from build123d import *

# Parameters (mm, degrees)
EXTRUDE_3_DEPTH          = 74.4
CUT_EXTRUDE_1_DEPTH      = 30
FILLET_1_R               = 5
CUT_EXTRUDE_6_DEPTH      = 330.484992071
CUT_EXTRUDE_6_DEPTH_BACK = 330.484992071
SKETCH_13_R              = 1.25
CUT_EXTRUDE_7_DEPTH      = 330.484992071
CUT_EXTRUDE_7_DEPTH_BACK = 330.484992071
SKETCH_14_R              = 2
SKETCH_15_R              = 2.5
CUT_EXTRUDE_8_DEPTH      = 100


with BuildPart() as part:
    # 草图4 → 凸台-拉伸3 (new body)
    with BuildSketch(Plane(origin=(0, 0, 0), x_dir=(0, 0, -1), z_dir=(1, 0, 0))):
        with BuildLine():
            Line((-19.997222801, -0.333287047), (-14.997222801, -300.333287047))
            ThreePointArc((-14.997222801, -300.333287047), (5.333287047, -319.997222801), (24.997222801, -299.666712953))
            Line((24.997222801, -299.666712953), (19.997222801, 0.333287047))
            ThreePointArc((19.997222801, 0.333287047), (-0.333287047, 19.997222801), (-19.997222801, -0.333287047))
        make_face()
    extrude(amount=EXTRUDE_3_DEPTH)

    # 草图8 → 切除-拉伸1 (cut)
    with BuildSketch(Plane(origin=(74.4, 0, 0), x_dir=(0, 0, -1), z_dir=(1, 0, 0))):
        with BuildLine():
            Line((-15.947486862, -243.317443397), (24.058068308, -243.317443397))
            Line((24.058068308, -243.317443397), (24.997222801, -299.666712953))
            ThreePointArc((24.997222801, -299.666712953), (4.858283924, -320.480273081), (-15.947486862, -300.333287047))
            Line((-15.947486862, -300.333287047), (-15.947486862, -243.317443397))
        make_face()
    extrude(amount=-CUT_EXTRUDE_1_DEPTH, mode=Mode.SUBTRACT)

    # 圆角1
    fillet_1_edges = [part.edges().sort_by_distance(p)[0] for p in [
        (74.4, -121.492078175, -22.027645554),
        (74.4, -243.317443397, -4.055290723),
        (74.4, 19.997222801, 0.333287047),
        (74.4, -121.825365222, 17.972354831),
    ]]
    fillet(fillet_1_edges, radius=FILLET_1_R)

    # 草图13 → 切除-拉伸6 (cut, two sides: drawn at the far end of the back side and taken through both)
    with BuildSketch(Plane.ZY.offset(-CUT_EXTRUDE_6_DEPTH_BACK)):
        with Locations(Location((-5.333287046, -270.358832161, 0), (0, 0, 180))):
            Circle(SKETCH_13_R)
        with Locations(Location((5.492030501, -276.608832161, 0), (0, 0, 180))):
            Circle(SKETCH_13_R)
        with Locations(Location((5.492030501, -289.108832161, 0), (0, 0, 180))):
            Circle(SKETCH_13_R)
        with Locations(Location((-5.333287046, -295.358832161, 0), (0, 0, 180))):
            Circle(SKETCH_13_R)
        with Locations(Location((-16.158604593, -289.108832161, 0), (0, 0, 180))):
            Circle(SKETCH_13_R)
        with Locations(Location((-16.158604593, -276.608832161, 0), (0, 0, 180))):
            Circle(SKETCH_13_R)
    extrude(amount=CUT_EXTRUDE_6_DEPTH + CUT_EXTRUDE_6_DEPTH_BACK, mode=Mode.SUBTRACT)

    # 草图14 → 切除-拉伸7 (cut, two sides: drawn at the far end of the back side and taken through both)
    with BuildSketch(Plane.ZY.offset(-CUT_EXTRUDE_7_DEPTH_BACK)):
        with Locations(Location((-5.333287046, -282.858832161, 0), (0, 0, 180))):
            Circle(SKETCH_14_R)
    extrude(amount=CUT_EXTRUDE_7_DEPTH + CUT_EXTRUDE_7_DEPTH_BACK, mode=Mode.SUBTRACT)

    # 草图15 → 切除-拉伸8 (cut)
    with BuildSketch(Plane.ZY):
        Circle(SKETCH_15_R)
    extrude(amount=-CUT_EXTRUDE_8_DEPTH, mode=Mode.SUBTRACT)


solid = part.part
The listing builds one solid part. Answer for the finished solid, in the listing's coordinates (mm). A direction names the side the tool comes from. Round coordinates to 2 decimals unless told otherwise and drop trailing zeros. Order: outer loops, then holes, each group sorted by start corner. A loop starts at its lowest first (then second) coordinate and runs counter-clockwise, first axis right, second up. Notation, with made-up numbers: (-32, 5) - (-15, 5) arc R22 cw to (-15, 27) - close; hole circle Ø3 at (78.25, 64). An arc over 180 degrees is marked (long way). Write item = value, one per line. Start each with the question number.
1) Given pin 1 (1.5 mm diameter, centred on y = -289.11, z = -16.16, fed in from +X); pin 2 (4 mm diameter, centred on x = 61, z = 9, fed in from -Y); pin 3 (3 mm diameter, centred on y = -270.36, z = -5.33, fed in from -X); pin 4 (1.5 mm diameter, centred on x = 34, z = 0.5, fed in from -Y), each flat-ended and moving along its own axis, determine where each tip first touches the part or whether it passes through.
2) For faces 1 (the flat face through (0, -148, -2)), 2 (the cylindrical face through (72.974, -123.501, 16.441)), 3 (the flat face through (57, -243.317, -4)), 4 (the cylindrical face through (72.97, -119.81, -20.5)), 5 (the flat face through (74.4, -110, -2)), determine the directions among +Z, -Z, +X, -X, +Y, -Y from which every point of the face is accessible in a straight line to the end or side of a thin tool.
3) Section B-B, the plane x = 5.5 is taken. Count the separate pieces of the cut face and the enclosed holes in it, plus the area to 3 significant figures.
4) Straight lines are drawn through the part: L1, parallel to X at y = -290.5, z = 3.5; L2, parallel to Y at x = 3, z = 6; L3, parallel to Y at x = 27.5, z = -16. For each, find the intervals that lie inside material, in ascending order.
5) Section A-A, the plane x = 61 is taken. Write down the section's boundary in (y, z), plus the area to 3 significant figures.
Results list:
q1.pin_1 = through
q1.pin_2 = -243.32
q1.pin_3 = 0
q1.pin_4 = -319.43
q2.face_1 = +Z, -Z, -X, +Y, -Y
q2.face_2 = +Z, +X, -Y
q2.face_3 = +Z, -Z, +X, -Y
q2.face_4 = -Z, +X, +Y
q2.face_5 = +Z, -Z, +X, +Y, -Y
q3.separate_pieces = 1
q3.enclosed_holes = 8
q3.area = 13,200 mm^2
q4.L1 = 0 to 44.4
q4.L2 = -316.7 to -290.25, -287.97 to -277.75, -275.47 to 19.08
q4.L3 = -316.7 to -290.35, -287.87 to -277.85, -275.37 to 12
q5.outline = (-243.32, -24.06) - (0.33, -20) arc R20 ccw to (-0.33, 20) - (-243.32, 15.95) - close; hole circle Ø5 at (0, 0)
q5.area = 10,300 mm^2
